from build123d import *

# Parameters (mm, degrees)
F1_W     = 127
F1_H     = 127
F2_DEPTH = 3.175
F3_DEPTH = 25.4
F5_DEPTH = 25.4


with BuildPart() as f2:
    # F1 (on Top) → F2 (new body)
    with BuildSketch(Plane.XY):
        Rectangle(F1_W, F1_H)
    extrude(amount=F2_DEPTH)

    # F0 (on Top) → F3 (cut)
    with BuildSketch(Plane.XY):
        Polygon((0, -39.167517), (32.015065, -20.683611), (30.110065, -19.583758), (0.9525, -36.417886), (0, -36.967812), (-0.9525, -36.417886), (-30.110065, -19.583758), (-32.015065, -20.683611), align=None)
        Polygon((30.110065, 19.583758), (32.015065, 20.683611), (0, 39.167517), (-32.015065, 20.683611), (-30.110065, 19.583758), (0, 36.967812), align=None)
        Polygon((33.920065, -19.583758), (33.920065, 19.583758), (32.015065, 18.483906), (0, 0), (-32.015065, 18.483906), (-33.920065, 19.583758), (-33.920065, -19.583758), (-32.015065, -18.483906), (-27.570065, -15.917584), (-27.570065, 6.385531), (-27.570065, 8.585236), (0, -7.332348), (27.570065, 8.585236), (27.570065, 6.385531), (27.570065, -15.917584), (32.015065, -18.483906), align=None)
        Polygon((0, -36.967812), (0.9525, -36.417886), (0.9525, -10.081979), (0, -9.532053), align=None)
        Polygon((-0.9525, -36.417886), (0, -36.967812), (0, -9.532053), (-0.9525, -10.081979), align=None)
    extrude(amount=F3_DEPTH, mode=Mode.SUBTRACT)

    # F4 (on face) → F5 (cut)
    with BuildSketch(Plane.XY.offset(3.175)):
        with BuildLine():
            ThreePointArc((-47.625, 44.45), (-45.379936, 45.379936), (-44.45, 47.625))
            Line((-44.45, 47.625), (-47.625, 47.625))
            Line((-47.625, 47.625), (-47.625, 44.45))
        make_face()
        with BuildLine():
            Line((-47.625, 47.625), (-44.45, 47.625))
            ThreePointArc((-44.45, 47.625), (-49.870064, 49.870064), (-47.625, 44.45))
            Line((-47.625, 44.45), (-47.625, 47.625))
        make_face()
        with BuildLine():
            ThreePointArc((50.8, -47.625), (49.870064, -45.379936), (47.625, -44.45))
            Line((47.625, -44.45), (47.625, -47.625))
            Line((47.625, -47.625), (44.45, -47.625))
            ThreePointArc((44.45, -47.625), (47.625, -50.8), (50.8, -47.625))
        make_face()
        with BuildLine():
            Line((47.625, -47.625), (47.625, -44.45))
            ThreePointArc((47.625, -44.45), (45.379936, -45.379936), (44.45, -47.625))
            Line((44.45, -47.625), (47.625, -47.625))
        make_face()
    extrude(amount=-F5_DEPTH, mode=Mode.SUBTRACT)


solid = f2.part
Read the model definition and answer for the solid it produces. Units are mm, in the model's axes. A direction names the side the tool comes from. Coordinates: 2 decimals unless noted, no trailing zeros. Loops run counter-clockwise (first coordinate to the right, second up) from the corner with the lowest first, then second, coordinate; pieces in that order, holes last.
Q1. The mould has two halves that part along Y. Classify faces 1 (the face through (-1, 63.5, 2)), 2 (the face through (27.57, -3, 2)), 3 (the face through (-1, -63.5, 2)): +Y half, -Y half, draft (parallel to the pull), parting line (faces both ways), or undercut.
Q2. The part is cut by section C-C on z = 1.7. Give the number of separate pieces and of enclosed holes in the cut face, and give its area (3 significant figures).
Q3. The part is cut by section A-A on y = 26. Write down the section's boundary in (x, z) (3 decimals).
Q4. Consider probe 1 along X at (y, z) = (-8, 0.75); probe 2 along Y at (x, z) = (0, 1.4); probe 3 along X at (y, z) = (28, 2.9). Determine where each line is inside the solid, lowest interval first.
Q5. Which of the six approach directions +Z, -Z, +X, -X, +Y, -Y give full straight-line access (tool end or side, diameter ignored) to faces 4 (the face through (15.783, -30.055, 1.565)), 5 (the face through (-63.5, -1, 2))?
Q6. The part is cut by section B-B on x = -16.5. Write down the section's boundary in (y, z) (3 decimals), and give its area (3 significant figures).
Results below:
1. face 1: +Y half
1. face 2: undercut
1. face 3: -Y half
2. separate pieces: 1
2. enclosed holes: 5
2. area: 14,900 mm2
3. outline: (-63.5, 0) - (-22.807, 0) - (-22.807, 3.175) - (-63.5, 3.175) - close; (-18.997, 0) - (18.997, 0) - (18.997, 3.175) - (-18.997, 3.175) - close; (22.807, 0) - (63.5, 0) - (63.5, 3.175) - (22.807, 3.175) - close
4. probe 1: x = -63.5 to -33.92, -27.57 to 27.57, 33.92 to 63.5
4. probe 2: y = -63.5 to -39.17, -9.53 to -7.33, 0 to 36.97, 39.17 to 63.5
4. probe 3: x = -63.5 to -19.34, -15.53 to 15.53, 19.34 to 63.5
5. face 4: +Z, -Z
5. face 5: +Z, -Z, -X, +Y, -Y
6. outline: (-63.5, 0) - (-29.641, 0) - (-29.641, 3.175) - (-63.5, 3.175) - close; (-27.442, 0) - (2.194, 0) - (2.194, 3.175) - (-27.442, 3.175) - close; (9.526, 0) - (27.442, 0) - (27.442, 3.175) - (9.526, 3.175) - close; (29.641, 0) - (63.5, 0) - (63.5, 3.175) - (29.641, 3.175) - close
6. area: 366 mm2
